Design review of the part built by this model. Coordinates are the model's own, in mm. A direction names the side the tool comes from. Round coordinates to 2 decimals unless told otherwise and drop trailing zeros. Order: outer loops, then holes, each group sorted by start corner. A loop starts at its lowest first (then second) coordinate and runs counter-clockwise, first axis right, second up. Notation, with made-up numbers: (73, 39) - (101, 39) arc R28 cw to (101, 61) - close; hole circle Ø4 at (-11.75, 59). An arc over 180 degrees is marked (long way). Write item = value, one per line.
from build123d import *

# Parameters (mm, degrees)
F1_DEPTH = 78
F2_R     = 6.5
F3_DEPTH = 25


with BuildPart() as f1:
    # F0 (on Front) → F1 (new body)
    with BuildSketch(Plane.XZ):
        with BuildLine():
            Line((0, 50.157899), (0, 88.157899))
            Line((0, 88.157899), (-7, 88.157899))
            Line((-7, 88.157899), (-7, 57.157899))
            ThreePointArc((-7, 57.157899), (-7.87868, 55.036578), (-10, 54.157899))
            Line((-10, 54.157899), (-65, 54.157899))
            ThreePointArc((-65, 54.157899), (-67.12132, 53.279219), (-68, 51.157899))
            Line((-68, 51.157899), (-68, 21.157899))
            ThreePointArc((-68, 21.157899), (-67.12132, 19.036578), (-65, 18.157899))
            Line((-65, 18.157899), (-10, 18.157899))
            ThreePointArc((-10, 18.157899), (-7.87868, 17.279219), (-7, 15.157899))
            Line((-7, 15.157899), (-7, -15.842101))
            Line((-7, -15.842101), (0, -15.842101))
            Line((0, -15.842101), (0, 22.157899))
            ThreePointArc((0, 22.157899), (-0.87868, 24.279219), (-3, 25.157899))
            Line((-3, 25.157899), (-58, 25.157899))
            ThreePointArc((-58, 25.157899), (-60.12132, 26.036578), (-61, 28.157899))
            Line((-61, 28.157899), (-61, 44.157899))
            ThreePointArc((-61, 44.157899), (-60.12132, 46.279219), (-58, 47.157899))
            Line((-58, 47.157899), (-3, 47.157899))
            ThreePointArc((-3, 47.157899), (-0.87868, 48.036578), (0, 50.157899))
        make_face()
    extrude(amount=F1_DEPTH)

    # F2 (on face) → F3 (cut)
    with BuildSketch(Plane(origin=(-7, 0, 0), x_dir=(0, -1, 0), z_dir=(-1, 0, 0))):
        with Locations((61.5, 74.157899)):
            Circle(F2_R)
        with Locations((16.5, 74.157899)):
            Circle(F2_R)
        with Locations((16.5, -1.842101)):
            Circle(F2_R)
        with Locations((61.5, -1.842101)):
            Circle(F2_R)
        Polygon((78, 88.157899), (68, 88.157899), (78, 78.157899), align=None)
        Polygon((0, 88.157899), (0, 78.157899), (10, 88.157899), align=None)
        Polygon((78, -5.842101), (68, -15.842101), (78, -15.842101), align=None)
        Polygon((0, -15.842101), (10, -15.842101), (0, -5.842101), align=None)
    extrude(amount=-F3_DEPTH, mode=Mode.SUBTRACT)


solid = f1.part
Item 1: Take a section at C-C, the plane y = -51. State the section outline as (x, z) points.
Data:
outline = (-68, 21.16) arc R3 ccw to (-65, 18.16) - (-10, 18.16) arc R3 cw to (-7, 15.16) - (-7, -15.84) - (0, -15.84) - (0, 22.16) arc R3 ccw to (-3, 25.16) - (-58, 25.16) arc R3 cw to (-61, 28.16) - (-61, 44.16) arc R3 cw to (-58, 47.16) - (-3, 47.16) arc R3 ccw to (0, 50.16) - (0, 88.16) - (-7, 88.16) - (-7, 57.16) arc R3 cw to (-10, 54.16) - (-65, 54.16) arc R3 ccw to (-68, 51.16) - close
Item 2: For line 1 along Z through (x, y) = (-34.5, -15); line 2 along Z through (x, y) = (-3, -16.5); line 3 along Z through (x, y) = (-2.5, -61.5), list the stretches that pass through material, from the lowest coordinate up. Write a range as [from, to].
Data:
line_1 = [18.16, 25.16], [47.16, 54.16]
line_2 = [-15.84, -8.34], [4.66, 25.16], [47.16, 67.66], [80.66, 88.16]
line_3 = [-15.84, -8.34], [4.66, 25.12], [47.2, 67.66], [80.66, 88.16]
Item 3: The part is to be moulded in two halves that separate along Z. For faces 3 (the face through (-38, -38, 18.158)), 4 (the face through (-61, -38, 36)), 5 (the face through (-7, -38, 73)), 6 (the face through (-7.855, -38.454, 55.06)), say which applies: +Z half, -Z half, draft (parallel to the pull), parting line (faces both ways), or undercut.
Data:
face_3 = -Z half
face_4 = undercut
face_5 = draft
face_6 = +Z half
Item 4: Insertion check: P1, Ø4, axis at x = -34.5, y = -40, coming from the -Z side; P2, Ø17.5, axis at y = -53, z = 39, coming from the +X side; P3, Ø2, axis at x = -24, y = -43, coming from the +Z side. Each pin has a flat end and moves straight along its axis. Give the tip position at first contact, or say it passes through.
Data:
P1 = 18.16
P2 = -1.21
P3 = 54.16
Item 5: Take a section at D-D, the plane z = 11. State the section outline as (x, y) points, and give its area (3 significant figures).
Data:
outline = (-7, -78) - (0, -78) - (0, 0) - (-7, 0) - close
area = 546 mm2
Item 6: Take a section at A-A, the plane y = -16.5. State the section outline as (x, z) points.
Data:
outline = (-68, 21.16) arc R3 ccw to (-65, 18.16) - (-10, 18.16) arc R3 cw to (-7, 15.16) - (-7, 4.66) - (0, 4.66) - (0, 22.16) arc R3 ccw to (-3, 25.16) - (-58, 25.16) arc R3 cw to (-61, 28.16) - (-61, 44.16) arc R3 cw to (-58, 47.16) - (-3, 47.16) arc R3 ccw to (0, 50.16) - (0, 67.66) - (-7, 67.66) - (-7, 57.16) arc R3 cw to (-10, 54.16) - (-65, 54.16) arc R3 ccw to (-68, 51.16) - close; (-7, -15.84) - (0, -15.84) - (0, -8.34) - (-7, -8.34) - close; (-7, 80.66) - (0, 80.66) - (0, 88.16) - (-7, 88.16) - close
Item 7: Take a section at B-B, the plane x = -22. State the section outline as (y, z) points, and give its area (3 significant figures).
Data:
outline = (-78, 18.16) - (0, 18.16) - (0, 25.16) - (-78, 25.16) - close; (-78, 47.16) - (0, 47.16) - (0, 54.16) - (-78, 54.16) - close
area = 1,090 mm2
Item 8: For faces 1 (the face through (-0.902, -38.454, 48.013)), 2 (the face through (-3.549, -67.504, 71.668)), list the 3-axis set-ups (+Z, -Z, +X, -X, +Y, -Y) from which the entire face can be reached by the end or side of a thin tool; tool diameter is ignored.
Data:
face_1 = +X, +Y, -Y
face_2 = +X, -X
